from build123d import *

# Parameters (mm, degrees)
SKETCH1_W                = 50
SKETCH1_H                = 15
BOSS_EXTRUDE1_DEPTH      = 2
SKETCH2_R                = 3.5
CUT_EXTRUDE1_DEPTH       = 2
SKETCH3_W                = 4
SKETCH3_H                = 15
BOSS_EXTRUDE2_DEPTH      = 4
SKETCH4_R                = 0.7
CUT_EXTRUDE2_DEPTH       = 67.866379361
M1_6X0_35_TAPPED_HOLE2_D = 1.25
M1_6X0_35_TAPPED_HOLE1_D = 1.25


with BuildPart() as part:
    # Sketch1 → Boss-Extrude1 (new body)
    with BuildSketch(Plane(origin=(0, 0, 0), x_dir=(1, 0, 0), z_dir=(0, 1, 0))):
        with Locations((-39.885381165, 7.155172414)):
            Rectangle(SKETCH1_W, SKETCH1_H)
    extrude(amount=BOSS_EXTRUDE1_DEPTH)

    # Sketch2 → Cut-Extrude1 (cut)
    with BuildSketch(Plane(origin=(0, 2, 0), x_dir=(1, 0, 0), z_dir=(0, 1, 0))):
        with Locations(Location((-39.885381165, 8.155172414, 0), (0, 0, 270))):
            Circle(SKETCH2_R)
    extrude(amount=-CUT_EXTRUDE1_DEPTH, mode=Mode.SUBTRACT)

    # Sketch3 → Boss-Extrude2 (add)
    with BuildSketch(Plane(origin=(0, 2, 0), x_dir=(1, 0, 0), z_dir=(0, 1, 0))):
        with Locations((-62.885381165, 7.155172414)):
            Rectangle(SKETCH3_W, SKETCH3_H)
        with Locations((-16.885381165, 7.155172414)):
            Rectangle(SKETCH3_W, SKETCH3_H)
    extrude(amount=BOSS_EXTRUDE2_DEPTH)

    # Sketch4 → Cut-Extrude2 (cut, through all)
    with BuildSketch(Plane(origin=(0, 0, -14.655172414), x_dir=(-1, 0, 0), z_dir=(0, 0, -1))):
        with Locations((62.885381165, 3)):
            Circle(SKETCH4_R)
        with Locations((16.885381165, 3)):
            Circle(SKETCH4_R)
    extrude(amount=-CUT_EXTRUDE2_DEPTH, mode=Mode.SUBTRACT)

    # M1.6x0.35 Tapped Hole2 (through all)
    with Locations(Plane(origin=(0, 2, 0), x_dir=(1, 0, 0), z_dir=(0, 1, 0))):
        with Locations((-44.885381165, 8.155172414)):
            Hole(M1_6X0_35_TAPPED_HOLE2_D / 2)

    # M1.6x0.35 Tapped Hole1 (through all)
    with Locations(Plane(origin=(0, 2, 0), x_dir=(1, 0, 0), z_dir=(0, 1, 0))):
        with Locations((-53.083792801, 8.155172414)):
            Hole(M1_6X0_35_TAPPED_HOLE1_D / 2)


solid = part.part
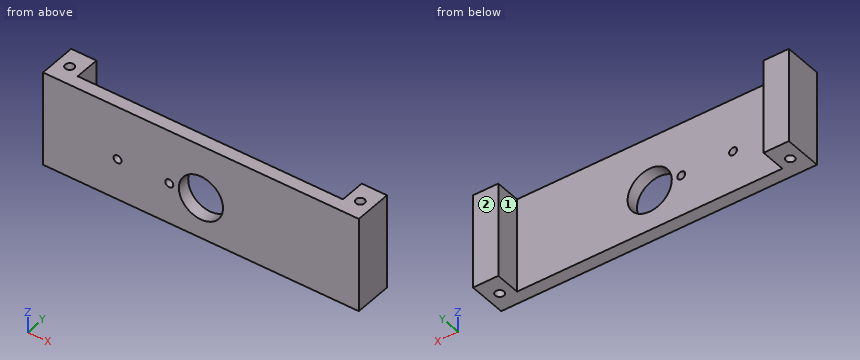
The listing builds one solid part. Answer for the finished solid, in the listing's coordinates (mm). Face numbers are marked on the shaded views. A direction names the side the tool comes from. Give positions to 0.01 mm unless a question says otherwise; leave off trailing zeros. Write each loop counter-clockwise with the first axis right and the second up, starting at its lowest first coordinate (ties: lowest second). Pieces come first, ordered by that corner, then holes. Notation, with made-up numbers: (29.25, 80.5) - (46.25, 80.5) arc R31 ccw to (46.25, 116.5) - close; hole circle Ø9 at (-39, 55). An arc over 180 degrees is marked (long way). Use a Markdown table: item, result.
1. Each of these flat-tipped pins is pushed along its axis until it touches: P1, Ø0.8, axis at x = -53.08, z = -8.16, coming from the -Y side; P2, Ø8, axis at x = -35, z = -11, coming from the +Y side. Where does it stop, or does it pass through?
Values follow:
| item | result |
|---|---|
| P1 | passes through |
| P2 | stops at y = 2 |
2. Section A-A on y = 4.85 is taken. Write down the section's boundary in (x, z), plus the area to 3 significant figures.
Values follow:
| item | result |
|---|---|
| outline | (-64.89, -14.66) - (-60.89, -14.66) - (-60.89, 0.34) - (-64.89, 0.34) - close; (-18.89, -14.66) - (-14.89, -14.66) - (-14.89, 0.34) - (-18.89, 0.34) - close |
| area | 120 mm² |
3. Section C-C on y = 3 is taken. Write down the section's boundary in (x, z), plus the area to 3 significant figures.
Values follow:
| item | result |
|---|---|
| outline | (-64.89, -14.66) - (-63.59, -14.66) - (-63.59, 0.34) - (-64.89, 0.34) - close; (-62.19, -14.66) - (-60.89, -14.66) - (-60.89, 0.34) - (-62.19, 0.34) - close; (-18.89, -14.66) - (-17.59, -14.66) - (-17.59, 0.34) - (-18.89, 0.34) - close; (-16.19, -14.66) - (-14.89, -14.66) - (-14.89, 0.34) - (-16.19, 0.34) - close |
| area | 78.0 mm² |
4. Section D-D on z = -2.5 is taken. Write down the section's boundary in (x, y), plus the area to 3 significant figures.
Values follow:
| item | result |
|---|---|
| outline | (-64.89, 0) - (-14.89, 0) - (-14.89, 6) - (-18.89, 6) - (-18.89, 2) - (-60.89, 2) - (-60.89, 6) - (-64.89, 6) - close; hole circle Ø1.4 at (-62.89, 3); hole circle Ø1.4 at (-16.89, 3) |
| area | 129 mm² |
5. A tool of negligible diameter and unlimited length cuts with its end or side. For the marked faces 1 and 2, from which of +Z, -Z, +X, -X, +Y, -Y can it reach the whole face along a straight path? Write none if from no direction.
Values follow:
| item | result |
|---|---|
| face 1 | +Z, -Z, +Y |
| face 2 | +Z, -Z, +X, -X, +Y |
6. Section B-B on z = -6 is taken. Write down the section's boundary in (x, y), plus the area to 3 significant figures.
Values follow:
| item | result |
|---|---|
| outline | (-64.89, 0) - (-42.64, 0) - (-42.64, 2) - (-60.89, 2) - (-60.89, 6) - (-64.89, 6) - close; (-37.13, 0) - (-14.89, 0) - (-14.89, 6) - (-18.89, 6) - (-18.89, 2) - (-37.13, 2) - close; hole circle Ø1.4 at (-62.89, 3); hole circle Ø1.4 at (-16.89, 3) |
| area | 118 mm² |
7. Find the intervals of material crossed by probe 1 along X at (y, z) = (4.8, -10.25); probe 2 along X at (y, z) = (2.4, -6.25); probe 3 along Y at (x, z) = (-31.5, -4), in increasing order. Write a range as from..to.
Values follow:
| item | result |
|---|---|
| probe 1 | x = -64.89..-60.89, -18.89..-14.89 |
| probe 2 | x = -64.89..-63.25, -62.52..-60.89, -18.89..-17.25, -16.52..-14.89 |
| probe 3 | y = 0..2 |
